Could you check a few things on this model? Use its own coordinates, in mm. Face numbers are marked on the shaded views. A direction names the side the tool comes from. Give positions to 0.01 mm unless a question says otherwise; leave off trailing zeros. Loops run counter-clockwise (first coordinate to the right, second up) from the corner with the lowest first, then second, coordinate; pieces in that order, holes last. Notation, with made-up numbers: (26, 28.5) - (83, 28.5) arc R14 ccw to (83, 32.5) - close; hole circle Ø7 at (27.5, 68). An arc over 180 degrees is marked (long way). Answer in a Markdown table with one row per item. Add a question column.
Autodesk Inventor part; units mm, degrees
ref_plane "Work Plane1" through (0, 0, 1.5) normal (0, 0, 1) x (1, 0, 0)
ref_plane "Work Plane2" through (-5, -9, 1.5) normal (0, -1, 0) x (1, 0, 0)
ref_plane "Work Plane3" through (-7.5, 0, 0) normal (1, 0, 0) x (0, 0, -1)
sketch "Sketch1" plane through (0, 0, 0) normal (1, 0, 0) x (0, 1, 0)
  circle A0 centre (0, 0) radius 9
  dimension "d31" = 18
extrude "Extrusion1" add sketch "Sketch1" against normal blind 15
hole "Hole1" at (0, 0, 0) direction (-1, 0, 0) diameter 13.5 end through all
ref_plane "Work Plane1" through (0, 0, 1.5) normal (0, 0, 1) x (1, 0, 0)
ref_plane "Work Plane2" through (-5, -9, 1.5) normal (0, -1, 0) x (1, 0, 0)
sketch "Sketch4" plane through (-5, -9, 1.5) normal (0, -1, 0) x (1, 0, 0)
  line L0 (-10, -3) -> (-5, -3)
  line L1 (-10, 0) -> (-10, -6) construction
  line L2 (-40.0446, 0) -> (21.4016, 0) construction
  line L3 (-5, 0) -> (-5, 0.1987) construction
  arc A0 (-10, -6) -> (-5.0454, -0.225) centre (-12.8638, 1.4698) ccw construction
  arc A1 (-5.0454, -0.225) -> (-5, 0.1987) centre (-7, 0.1987) ccw construction
  line L4 (-10, -3) -> (-10, 3)
  line L5 (-5, -3) -> (-5, -0.7378)
  arc A2 (-5.5557, 0.6457) -> (-10, 3) centre (-11.3329, -4.8882) ccw
  arc A3 (-5, -0.7378) -> (-5.5557, 0.6457) centre (-7, -0.7378) ccw
  line L6 (-10, -8.25) -> (-10, 5.25) construction
  line L7 (-10, -8.25) -> (-10, 5.25) construction
  line L8 (-10, 7.5) -> (-10, -10.5) construction
  line L9 (-10, 7.5) -> (12.6236, 7.5)
  line L10 (-5, -1.5) -> (12.6236, -1.5)
  line L11 (-10, 7.5) -> (5, 7.5)
  line L12 (-2.5, 7.5) -> (-2.5, -13.092)
  line L13 (35.0446, 0) -> (-26.4016, 0) construction
  arc A4 (0.0454, -0.225) -> (5, -6) centre (7.8638, 1.4698) ccw construction
  arc A5 (0.0099, 0) -> (0.0454, -0.225) centre (2, 0.1987) ccw
  line L14 (5, 0.1987) -> (5, -10.5) construction
  line L15 (5, -6) -> (5, 0) construction
  line L16 (0.0099, 0) -> (5, 0) construction
  line L17 (-10, 3) -> (6.7233, 3)
  arc A6 (0.0099, -3) -> (0.0454, -3.225) centre (2, -2.8013) ccw
  arc A7 (0.0454, -3.225) -> (5, -9) centre (7.8638, -1.5302) ccw
  line L18 (5, -9) -> (5, -3)
  line L19 (0.0099, -3) -> (5, -3)
  line L20 (-10, -3) -> (-5, -3)
  line L21 (0.0099, -3) -> (12.6236, -3)
  point P0 (5, -1.5)
  point P1 (-4.9623, 0.2185)
  point P2 (-5, 0)
  point P3 (-4.9623, -0.2185)
  point P4 (-5, 0)
  point P5 (-0.0377, 0.2185)
  point P6 (0, 0)
  point P7 (-0.0377, -0.2185)
  point P8 (0, 0)
  point P9 (5, 0)
  dimension "d43" = 6
  dimension "d47" = 2
  dimension "d49" = 8
  dimension "d76" = 18
  dimension "d77" = 9
  dimension "d78" = 6
  dimension "d79" = 8
  dimension "d80" = 2
  dimension "d81" = 5
  dimension "d82" = 1.5
  dimension "d84" = 15
extrude "Extrusion7" cut sketch "Sketch4" against normal blind 10 contours L4 A2 A3 L5 L0 | L19 L18 A7 A6
pattern_circular "Circular Pattern3" count 6 over 360 about axis through (-10, 0, 0) along (1, 0, 0) of "Extrusion7"
ref_plane "Work Plane3" through (-7.5, 0, 0) normal (1, 0, 0) x (0, 0, -1)
sketch "Sketch6" plane through (-15, 0, 0) normal (-1, 0, 0) x (0, 0, 1)
  line L0 (-6.9352, 5.7361) -> (1.5, 8.8741)
  line L1 (6.9352, -5.7361) -> (4.9495, -4.5896) construction
  line L2 (4.5, -5.0312) -> (4.5, -7.7942) construction
  arc A0 (4.5, -7.7942) -> (6.9352, -5.7361) centre (0, 0) ccw construction
  line L3 (8.4352, 3.138) -> (6.4495, 1.9916) construction
  line L4 (6.6071, 1.3815) -> (9, 0) construction
  arc A1 (9, 0) -> (8.4352, 3.138) centre (0, 0) ccw construction
  line L5 (2.1071, 6.4127) -> (4.5, 7.7942) construction
  arc A2 (4.5, 7.7942) -> (1.5, 8.8741) centre (0, 0) ccw construction
  line L6 (1.5, 8.8741) -> (1.5, 6.5812) construction
  line L7 (-4.5, 5.0312) -> (-4.5, 7.7942) construction
  arc A3 (-4.5, 7.7942) -> (-6.9352, 5.7361) centre (0, 0) ccw construction
  line L8 (-6.9352, 5.7361) -> (-4.9495, 4.5896) construction
  line L9 (-6.6071, -1.3815) -> (-9, 0) construction
  arc A4 (-9, 0) -> (-8.4352, -3.138) centre (0, 0) ccw construction
  line L10 (-8.4352, -3.138) -> (-6.4495, -1.9916) construction
  line L11 (-2.1071, -6.4127) -> (-4.5, -7.7942) construction
  arc A5 (-4.5, -7.7942) -> (-1.5, -8.8741) centre (0, 0) ccw construction
  line L12 (-1.5, -8.8741) -> (-1.5, -6.5812) construction
  line L13 (0, 0) -> (-6.9352, 5.7361)
  line L14 (1.5, 8.8741) -> (0, 0)
  circle A6 centre (0, 0) radius 9
  line L15 (-8.4352, -3.138) -> (-6.9352, 5.7361)
  line L16 (0, 0) -> (-8.4352, -3.138)
  line L17 (-6.9352, 5.7361) -> (0, 0)
  line L18 (-1.5, -8.8741) -> (-8.4352, -3.138)
  line L19 (0, 0) -> (-1.5, -8.8741)
  line L20 (-8.4352, -3.138) -> (0, 0)
  line L21 (6.9352, -5.7361) -> (-1.5, -8.8741)
  line L22 (0, 0) -> (6.9352, -5.7361)
  line L23 (-1.5, -8.8741) -> (0, 0)
  line L24 (8.4352, 3.138) -> (6.9352, -5.7361)
  line L25 (0, 0) -> (8.4352, 3.138)
  line L26 (6.9352, -5.7361) -> (0, 0)
  line L27 (1.5, 8.8741) -> (8.4352, 3.138)
  line L28 (0, 0) -> (1.5, 8.8741)
  line L29 (8.4352, 3.138) -> (0, 0)
  arc A7 (-2.1071, -6.4127) -> (-1.5, -6.5812) centre (0, 0) ccw
  arc A8 (-6.6071, -1.3815) -> (-6.4495, -1.9916) centre (0, 0) ccw
  arc A9 (-4.5, 5.0312) -> (-4.9495, 4.5896) centre (0, 0) ccw
  arc A10 (2.1071, 6.4127) -> (1.5, 6.5812) centre (0, 0) ccw
  arc A11 (6.6071, 1.3815) -> (6.4495, 1.9916) centre (0, 0) ccw
  arc A12 (4.5, -5.0312) -> (4.9495, -4.5896) centre (0, 0) ccw
  dimension "d72" = 360
extrude "Extrusion11" cut sketch "Sketch6" against normal through all contours A6 L0 | L15 A6 | A6 L27 | L18 A6 | A6 L24 | L21 A6
properties part number "SPRING NUT1" material "Steel, Mild"
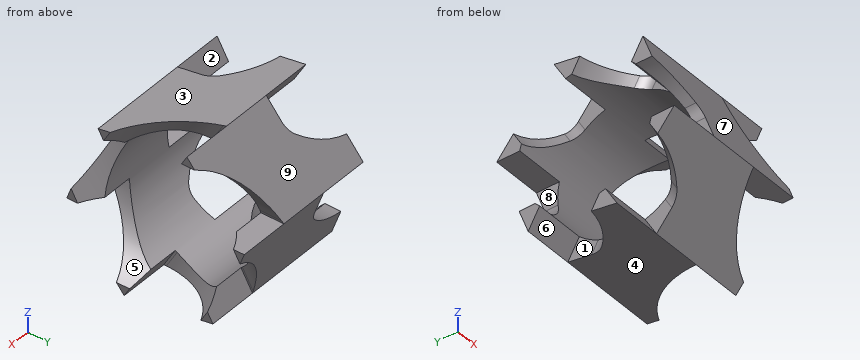
(1) On a 3-axis mill with a long thin cutter (end or side, diameter ignored), from which of +Z, -Z, +X, -X, +Y, -Y can I reach the whole of each face in a straight line? I mean the marked faces 5, 6, 7, 8 and 9. Say none if no direction works.
(2) Please list where these lines run through material, in increasing order: line 1 (Z direction, x = -10.25, y = 0); line 2 (Y direction, x = -6, z = 0); line 3 (Z direction, x = -5.5, y = -1).
(3) For pin 1 Ø2 at (y, z) = (-4, -7) entering from -X; pin 2 Ø1 at (y, z) = (1, 6.5) entering from +X; pin 3 Ø1.5 at (x, y) = (-6.5, 4) entering from -Z, each with a flat end and sliding along its axis, tell me the tip position at first contact or that it passes through.
(4) I want a section at A-A on x = -1.5. Please give me the cut outline in (y, z), then the cut area to 3 significant figures.
(5) We'd pull the mould along Y, two halves only. Please class the marked faces 1, 2, 3 and 4: pulls with the +Y half, pulls with the -Y half, needs draft (parallel to the pull), parting line crosses it, or undercut.
(6) I want a section at B-B on x = -8.75. Please give me the cut outline in (y, z).
Reported:
| question | item | result |
|---|---|---|
| 1 | face 5 | +X, -Y |
| 1 | face 6 | -Z, -X |
| 1 | face 7 | +Z, +X, -X, -Y |
| 1 | face 8 | -X, +Y |
| 1 | face 9 | +Z, +X, -X, +Y |
| 2 | line 1 | -7.9 to -6.75, 6.75 to 7.9 |
| 2 | line 2 | -8.32 to -6.75, 6.75 to 8.32 |
| 2 | line 3 | -8.07 to -6.68, 6.68 to 7.74 |
| 3 | pin 1 | x = -10.01 |
| 3 | pin 2 | x = -4.61 |
| 3 | pin 3 | z = -7.36 |
| 4 | outline | (-8.87, -1.5) - (-6.91, -1.5) - (-8.1, 0.57) - close; (-5.74, 6.94) - (-4.75, 5.24) - (-3.56, 7.3) - close; (-4.54, -6.74) - (-3.14, -8.44) - (-2.16, -6.74) - close; (2.16, 6.74) - (4.54, 6.74) - (3.14, 8.44) - close; (3.56, -7.3) - (5.74, -6.94) - (4.75, -5.24) - close; (6.91, 1.5) - (8.1, -0.57) - (8.87, 1.5) - close |
| 4 | area | 12.2 mm² |
| 5 | face 1 | undercut |
| 5 | face 2 | undercut |
| 5 | face 3 | pulls with the -Y half |
| 5 | face 4 | pulls with the +Y half |
| 6 | outline | (-8.87, -1.5) - (-3.14, -8.44) - (5.74, -6.94) - (8.87, 1.5) - (3.14, 8.44) - (-5.74, 6.94) - close; hole circle Ø13.5 at (0, 0) |
